```python
from build123d import *

# Parameters (mm, degrees)
F1_DEPTH             = 3
F2_W                 = 10
F2_H                 = 10
F3_DEPTH             = 5
F5_W                 = 10
F5_H                 = 10
F6_DEPTH             = 10
F8_D                 = 2.5
F8_DEPTH             = 5
F8_CSINK_D           = 4
F8_CSINK_ANGLE       = 90
F8_TIP               = 0.7510757738
F8_ON_F4_D           = 2.5
F8_ON_F4_DEPTH       = 5
F8_ON_F4_CSINK_D     = 4
F8_ON_F4_CSINK_ANGLE = 90
F8_ON_F4_TIP         = 0.7510757738
F9_W                 = 9
F9_H                 = 140
F10_DEPTH            = 11.5
F11_W                = 4.5
F11_H                = 140
F12_DEPTH            = 8
F14_DEPTH            = 19.5
F15_W                = 151
F15_H                = 7.5
F16_DEPTH            = 5
F18_DEPTH            = 3
F19_W                = 13
F19_H                = 10
F19_W_2              = 10
F20_DEPTH            = 5
F22_DEPTH            = 3
F23_W                = 13
F23_H                = 10
F24_DEPTH            = 15
F25_W                = 90
F25_H                = 15
F26_DEPTH            = 19.5
F27_SIZE             = 0.49999


# Not quite as in the source:
# - a fillet or chamfer is up to 0.001 mm smaller than in the source, because OpenCascade refuses the exact size
# - a feature names something its author has since deleted; it is built from what else it names


with BuildPart() as f1:
    # F0 (on Top) → F1 (new body)
    with BuildSketch(Plane.XY):
        with BuildLine():
            Line((-78, -75), (78, -75))
            ThreePointArc((78, -75), (79.4142135624, -74.4142135624), (80, -73))
            Line((80, -73), (80, 73))
            ThreePointArc((80, 73), (79.4142135624, 74.4142135624), (78, 75))
            Line((78, 75), (-78, 75))
            ThreePointArc((-78, 75), (-79.4142135624, 74.4142135624), (-80, 73))
            Line((-80, 73), (-80, -73))
            ThreePointArc((-80, -73), (-79.4142135624, -74.4142135624), (-78, -75))
        make_face()
    extrude(amount=F1_DEPTH)

    # F2 (on face) → F3 (join)
    with BuildSketch(Plane.XY.offset(3)):
        with Locations((-63, -40)):
            Rectangle(F2_W, F2_H)
        with Locations((-63, 50)):
            Rectangle(F2_W, F2_H)
        with Locations((63, 50)):
            Rectangle(F2_W, F2_H)
        with Locations((63, -40)):
            Rectangle(F2_W, F2_H)
    extrude(amount=F3_DEPTH)

    # F5 (on face) → F6 (join)
    with BuildSketch(Plane.XY.offset(3)):
        with Locations((-63, 60)):
            Rectangle(F5_W, F5_H)
        with Locations((-63, -50)):
            Rectangle(F5_W, F5_H)
        with Locations((63, 60)):
            Rectangle(F5_W, F5_H)
        with Locations((63, -50)):
            Rectangle(F5_W, F5_H)
    extrude(amount=F6_DEPTH)

    # F8
    with Locations(Plane.XY.offset(13)):
        with Locations((-63, 60), (63, 60)):
            CounterSinkHole(F8_D / 2, F8_CSINK_D / 2, depth=F8_DEPTH, counter_sink_angle=F8_CSINK_ANGLE)
            with Locations((0, 0, -(F8_DEPTH + F8_TIP / 2))):  # 118° drill point
                Cone(0, F8_D / 2, F8_TIP, mode=Mode.SUBTRACT)

    # F8 on F4
    with Locations(Plane.XY.offset(8)):
        with Locations((-63, -40), (63, -40), (-63, 50), (63, 50)):
            CounterSinkHole(F8_ON_F4_D / 2, F8_ON_F4_CSINK_D / 2, depth=F8_ON_F4_DEPTH, counter_sink_angle=F8_ON_F4_CSINK_ANGLE)
            with Locations((0, 0, -(F8_ON_F4_DEPTH + F8_ON_F4_TIP / 2))):  # 118° drill point
                Cone(0, F8_ON_F4_D / 2, F8_ON_F4_TIP, mode=Mode.SUBTRACT)

    # F9 (on face) → F10 (join)
    with BuildSketch(Plane.XY.offset(3)):
        with Locations((-75.5, 0)):
            Rectangle(F9_W, F9_H)
        with Locations((75.5, 0)):
            Rectangle(F9_W, F9_H)
    extrude(amount=F10_DEPTH)

    # F11 (on face) → F12 (join)
    with BuildSketch(Plane.XY.offset(14.5)):
        with Locations((-77.75, 0)):
            Rectangle(F11_W, F11_H)
        with Locations((77.75, 0)):
            Rectangle(F11_W, F11_H)
    extrude(amount=F12_DEPTH)

    # F13 (on face) → F14 (join, through all)
    with BuildSketch(Plane.XY.offset(3)):
        with BuildLine():
            Line((-80, -70), (-80, -73))
            ThreePointArc((-80, -73), (-79.4142135624, -74.4142135624), (-78, -75))
            Line((-78, -75), (78, -75))
            ThreePointArc((78, -75), (79.4142135624, -74.4142135624), (80, -73))
            Line((80, -73), (80, -70))
            Line((80, -70), (-80, -70))
        make_face()
        with BuildLine():
            Line((-80, 73), (-80, 70))
            Line((-80, 70), (80, 70))
            Line((80, 70), (80, 73))
            ThreePointArc((80, 73), (79.4142135624, 74.4142135624), (78, 75))
            Line((78, 75), (-78, 75))
            ThreePointArc((-78, 75), (-79.4142135624, 74.4142135624), (-80, 73))
        make_face()
    extrude(amount=F14_DEPTH)

    # F15 (on face) → F16 (cut, through all)
    with BuildSketch(Plane.XZ.offset(75)):
        with Locations((0, 18.25)):
            Rectangle(F15_W, F15_H)
    extrude(amount=-F16_DEPTH, mode=Mode.SUBTRACT)

    # F17 (on face) → F18 (join, through all)
    with BuildSketch(Plane(origin=(-68, 0, 0), x_dir=(0, -1, 0), z_dir=(-1, 0, 0))):
        Polygon((-65, 3), (-45, 3), (-45, 8), (-55, 8), (-55, 13), (-65, 13), align=None)
        Polygon((35, 3), (55, 3), (55, 13), (45, 13), (45, 8), (35, 8), align=None)
    extrude(amount=F18_DEPTH)

    # F19 (on face) → F20 (join, through all)
    with BuildSketch(Plane(origin=(0, 65, 0), x_dir=(-1, 0, 0), z_dir=(0, 1, 0))):
        with Locations((64.5, 8)):
            Rectangle(F19_W, F19_H)
        with Locations((-63, 8)):
            Rectangle(F19_W_2, F19_H)
    extrude(amount=F20_DEPTH)

    # F21 (on face) → F22 (join, through all)
    with BuildSketch(Plane.YZ.offset(68)):
        Polygon((45, 8), (45, 3), (70, 3), (70, 13), (55, 13), (55, 8), align=None)
        Polygon((-55, 13), (-55, 3), (-35, 3), (-35, 8), (-45, 8), (-45, 13), align=None)
    extrude(amount=F22_DEPTH)

    # F23 (on face) → F24 (join, through all)
    with BuildSketch(Plane.XZ.offset(55)):
        with Locations((64.5, 8)):
            Rectangle(F23_W, F23_H)
        with Locations((-64.5, 8)):
            Rectangle(F23_W, F23_H)
    extrude(amount=F24_DEPTH)

    # F25 (on face) → F26 (join, through all)
    with BuildSketch(Plane.XY.offset(3)):
        with Locations((0, 62.5)):
            Rectangle(F25_W, F25_H)
    extrude(amount=F26_DEPTH)

    # F27 (size 0.5 in the source; OpenCascade refuses exactly that, so slightly less here)
    f27_edges = [f1.edges().sort_by_distance(p)[0] for p in [
        (71, 0, 14.5),
        (-71, 0, 14.5),
        (-58, 62.5, 13),
        (-64.5, 55, 13),
        (-58, 50, 8),
        (-64.5, 45, 8),
        (-64.5, -45, 13),
        (-58, -40, 8),
        (-64.5, -35, 8),
        (58, 62.5, 13),
        (64.5, 55, 13),
        (58, 50, 8),
        (64.5, 45, 8),
        (-75.5, -75, 18.25),
        (0, -75, 14.5),
        (0, -75, 22),
        (75.5, -75, 18.25),
    ]]
    chamfer(f27_edges, length=F27_SIZE)


solid = f1.part
```
For this review, take the finished solid that the model builds, in its own axes (mm). Coordinates: 2 decimals unless noted, no trailing zeros. Loops run counter-clockwise (first coordinate to the right, second up) from the corner with the lowest first, then second, coordinate; pieces in that order, holes last. Notation, with made-up numbers: (32, -13.75) - (36, -13.75) arc R22 ccw to (36, 8.25) - close; hole circle Ø9 at (21, -29). An arc over 180 degrees is marked (long way). Use one line per item in the form item = value. Start each with the question number.
1) Take a section at D-D (y = -2.5). State the section outline as (x, z) points.
2) Take a section at B-B (y = -49.5). State the section outline as (x, z) points, plus the area to 3 significant figures.
3) For pin 1 (14.5 mm diameter, centred on x = -66.5, y = -54.5, fed in from +Z); pin 2 (7.5 mm diameter, centred on x = 62, y = 48, fed in from +Z); pin 3 (10 mm diameter, centred on x = 9, y = 26, fed in from +Z), all flat-tipped, find the tip position at first contact; note any pin that passes through.
4) Draft analysis for pull direction Y (two halves, no side actions). For faces 1 (the face through (80, -1, 11)), 2 (the face through (65, 51, 8)), 3 (the face through (65, 63, 13)), state which applies: released by +Y, released by -Y, zero draft, split by the parting line, or undercut.
5) To check wall thickness, follow probe 1 along Y at (x, z) = (-63, 4.65); probe 2 along X at (y, z) = (50, 4.8); probe 3 along X at (y, z) = (60, 10.5). State the ranges of each line that lie inside material, in increasing order. Write a range as from..to.
From the geometry:
q1.outline = (-80, 0) - (80, 0) - (80, 22.5) - (75.5, 22.5) - (75.5, 14.5) - (71.5, 14.5) - (71, 14) - (71, 3) - (-71, 3) - (-71, 14) - (-71.5, 14.5) - (-75.5, 14.5) - (-75.5, 22.5) - (-80, 22.5) - close
q2.outline = (-80, 0) - (80, 0) - (80, 22.5) - (75.5, 22.5) - (75.5, 14.5) - (71.5, 14.5) - (71, 14) - (71, 13) - (58, 13) - (58, 3) - (-58, 3) - (-58, 13) - (-71, 13) - (-71, 14) - (-71.5, 14.5) - (-75.5, 14.5) - (-75.5, 22.5) - (-80, 22.5) - close
q2.area = 1,020 mm2
q3.pin_1 = 14.5
q3.pin_2 = 8
q3.pin_3 = 3
q4.face_1 = zero draft
q4.face_2 = undercut
q4.face_3 = undercut
q5.probe_1 = -75..-41.25, -38.75..-35, 45..48.75, 51.25..75
q5.probe_2 = -80..-64.25, -61.75..-58, 58..61.75, 64.25..80
q5.probe_3 = -80..-64.25, -61.75..-58, -45..45, 58..61.75, 64.25..80
